Could you check a few things on this model? Use its own coordinates, in mm. A direction names the side the tool comes from. Give positions to 0.01 mm unless a question says otherwise; leave off trailing zeros. Write each loop counter-clockwise with the first axis right and the second up, starting at its lowest first coordinate (ties: lowest second). Pieces come first, ordered by that corner, then holes. Notation, with made-up numbers: (66.5, 59.25) - (70.5, 59.25) arc R9 ccw to (70.5, 74.25) - close; hole circle Ø9 at (10, 63). An arc over 180 degrees is marked (long way). Answer in a Markdown table with one row per item.
from build123d import *

# Parameters (mm, degrees)
BOX003_W          = 15
BOX003_H          = 15
BOX003_DEPTH      = 58
FILLET_R          = 10
CYLINDER_R        = 1
CYLINDER_DEPTH    = 58
CYLINDER001_R     = 1
CYLINDER001_DEPTH = 58
BOX002_W          = 10
BOX002_H          = 15
BOX002_DEPTH      = 58
BOX001_W          = 15
BOX001_H          = 10
BOX001_DEPTH      = 58
BOX_W             = 30
BOX_H             = 30
BOX_DEPTH         = 58
FILLET001_R       = 0.4


with BuildPart() as fillet_body:
    # Box003 → Box003 (new body)
    with BuildSketch(Plane(origin=(15, 15, 0), x_dir=(1, 0, 0), z_dir=(0, 0, 1))):
        with Locations((7.5, 7.5)):
            Rectangle(BOX003_W, BOX003_H)
    extrude(amount=BOX003_DEPTH)

    # Fillet
    fillet_edges = [fillet_body.edges().sort_by_distance(p)[0] for p in [
        (15, 15, 29),
    ]]
    fillet(fillet_edges, radius=FILLET_R)


with BuildPart() as cylinder:
    # Cylinder → Cylinder (new body)
    with BuildSketch(Plane(origin=(15, 10, 0), x_dir=(1, 0, 0), z_dir=(0, 0, 1))):
        Circle(CYLINDER_R)
    extrude(amount=CYLINDER_DEPTH)


with BuildPart() as cylinder001:
    # Cylinder001 → Cylinder001 (new body)
    with BuildSketch(Plane(origin=(10, 15, 0), x_dir=(1, 0, 0), z_dir=(0, 0, 1))):
        Circle(CYLINDER001_R)
    extrude(amount=CYLINDER001_DEPTH)


with BuildPart() as cube002:
    # Box002 → Box002 (new body)
    with BuildSketch(Plane(origin=(0, 15, 0), x_dir=(1, 0, 0), z_dir=(0, 0, 1))):
        with Locations((5, 7.5)):
            Rectangle(BOX002_W, BOX002_H)
    extrude(amount=BOX002_DEPTH)


with BuildPart() as cube001:
    # Box001 → Box001 (new body)
    with BuildSketch(Plane(origin=(15, 0, 0), x_dir=(1, 0, 0), z_dir=(0, 0, 1))):
        with Locations((7.5, 5)):
            Rectangle(BOX001_W, BOX001_H)
    extrude(amount=BOX001_DEPTH)


with BuildPart() as fillet001:
    # Box → Box (new body)
    with BuildSketch(Plane.XY):
        with Locations((15, 15)):
            Rectangle(BOX_W, BOX_H)
    extrude(amount=BOX_DEPTH)

    # Cut: cut Cube001
    add(cube001.part, mode=Mode.SUBTRACT)

    # Cut001: cut Cube002
    add(cube002.part, mode=Mode.SUBTRACT)

    # Cut002: cut Cylinder001
    add(cylinder001.part, mode=Mode.SUBTRACT)

    # Cut003: cut Cylinder
    add(cylinder.part, mode=Mode.SUBTRACT)

    # Cut004: cut Fillet body
    add(fillet_body.part, mode=Mode.SUBTRACT)

    # Fillet001
    fillet001_edges = [fillet001.edges().sort_by_distance(p)[0] for p in [
        (0, 15, 29),
        (0, 0, 29),
        (15, 0, 29),
        (15, 30, 29),
        (10, 30, 29),
        (30, 15, 29),
        (30, 10, 29),
    ]]
    fillet(fillet001_edges, radius=FILLET001_R)


solid = fillet001.part
1) If I drill on line 1 (Y direction, x = 6, z = 21.5); line 2 (X direction, y = 25.5, z = 17.5), over which ranges is the centre line in solid material (lowest first)?
Check values:
| item | result |
|---|---|
| line 1 | y = 0 to 15 |
| line 2 | x = 10 to 15 |
2) Will these pins go through, and if not, where does the flat tip stop? P1, Ø5, axis at x = 27.5, z = 16, coming from the +Y side; P2, Ø1.4, axis at y = 28.5, z = 31.5, coming from the +X side; P3, Ø11, axis at y = 22.5, z = 18, coming from the -X side.
Check values:
| item | result |
|---|---|
| P1 | stops at y = 15 |
| P2 | stops at x = 15 |
| P3 | stops at x = 10 |
3) Imagine slicing it at B-B (y = 6.25). List the corners of the cut face in (x, z) for me.
Check values:
| item | result |
|---|---|
| outline | (0, 0) - (15, 0) - (15, 58) - (0, 58) - close |
4) Imagine slicing it at A-A (z = 48.5). List the corners of the cut face in (x, y) for me.
Check values:
| item | result |
|---|---|
| outline | (0, 0.4) arc R0.4 ccw to (0.4, 0) - (14.6, 0) arc R0.4 ccw to (15, 0.4) - (15, 9) arc R1 cw (long way) to (16, 10) - (29.6, 10) arc R0.4 ccw to (30, 10.4) - (30, 14.6) arc R0.4 ccw to (29.6, 15) - (25, 15) arc R10 cw to (15, 25) - (15, 29.6) arc R0.4 ccw to (14.6, 30) - (10.4, 30) arc R0.4 ccw to (10, 29.6) - (10, 16) arc R1 cw (long way) to (9, 15) - (0.4, 15) arc R0.4 ccw to (0, 14.6) - close |
5) We'd pull the mould along X, two halves only. Please class faces 6 (the face through (14.317, 10.73, 28.594)), 7 (the face through (10, 23, 29)), 8 (the face through (23, 10, 29)), 9 (the face through (10.683, 14.27, 28.594)): +X half, -X half, draft (parallel to the pull), parting line (faces both ways), or undercut.
Check values:
| item | result |
|---|---|
| face 6 | undercut |
| face 7 | -X half |
| face 8 | draft |
| face 9 | undercut |
6) On a 3-axis mill with a long thin cutter (end or side, diameter ignored), from which of +Z, -Z, +X, -X, +Y, -Y can I reach the whole of each face in a straight line? I mean faces 1 (the face through (11, 12, 58)), 2 (the face through (5, 15, 29)), 3 (the face through (7, 0, 29)), 4 (the face through (15, 27, 29)), 5 (the face through (15, 5, 29)). Say none if no direction works.
Check values:
| item | result |
|---|---|
| face 1 | +Z, +X, -X, +Y, -Y |
| face 2 | +Z, -Z, -X, +Y |
| face 3 | +Z, -Z, +X, -X, -Y |
| face 4 | +Z, -Z, +X, +Y |
| face 5 | +Z, -Z, +X, -Y |
